from build123d import *

# Parameters (mm, degrees)
SKETCH1_R             = 10.5
SKETCH1_R_2           = 3
EXTRUDE1_DEPTH        = 46.5
SKETCH1_3_R           = 3
CUT_EXTRUDE1_DEPTH    = 49.813420286
CUT_EXTRUDE4_DEPTH    = 8.5
CUT_EXTRUDE6_START    = -37
SKETCH6_R             = 10.5
SKETCH6_R_2           = 6
CUT_EXTRUDE6_DEPTH    = 37
CUT_EXTRUDE7_START    = -1
SKETCH7_R             = 10.5
SKETCH7_R_2           = 7.5
CUT_EXTRUDE7_DEPTH    = 1
M4X0_7_TAPPED_HOLE1_D = 3
SKETCH8_OUTSIDE_W     = 33.82
SKETCH8_OUTSIDE_H     = 30.82
CUT_EXTRUDE8_DEPTH    = 30
FILLET1_R             = 0.5
CHAMFER1_SIZE         = 0.5
FILLET2_R             = 0.3
CHAMFER2_SIZE         = 1
SKETCH13_R            = 14.541098745
CUT_EXTRUDE9_DEPTH    = 9


with BuildPart() as part:
    # Sketch1 → Extrude1 (new body)
    # profile 1 of 2: a face of its own
    with BuildSketch(Plane.XY):
        Circle(SKETCH1_R)
        Circle(SKETCH1_R_2, mode=Mode.SUBTRACT)
    # profile 2 of 2: a face of its own
    with BuildSketch(Plane.XY):
        Circle(SKETCH1_R_2)
    extrude(amount=-EXTRUDE1_DEPTH)

    # Sketch1<3> → Cut-Extrude1 (cut, through all)
    with BuildSketch(Plane.XY):
        Circle(SKETCH1_3_R)
    extrude(amount=-CUT_EXTRUDE1_DEPTH, mode=Mode.SUBTRACT)

    # Sketch4 → Cut-Extrude4 (cut)
    with BuildSketch(Plane.XY):
        with BuildLine():
            Line((-10.24499878, 2.3), (10.24499878, 2.3))
            ThreePointArc((10.24499878, 2.3), (0, 10.5), (-10.24499878, 2.3))
        make_face()
    extrude(amount=-CUT_EXTRUDE4_DEPTH, mode=Mode.SUBTRACT)

    # Sketch6 → Cut-Extrude6 (cut)
    with BuildSketch(Plane(origin=(0, 0, -46.5), x_dir=(1, 0, 0), z_dir=(0, 0, -1)).offset(CUT_EXTRUDE6_START)):
        Circle(SKETCH6_R)
        with Locations(Location((0, 0, 0), (0, 0, 270))):
            Circle(SKETCH6_R_2, mode=Mode.SUBTRACT)
    extrude(amount=CUT_EXTRUDE6_DEPTH, mode=Mode.SUBTRACT)

    # Sketch7 → Cut-Extrude7 (cut)
    with BuildSketch(Plane(origin=(0, 0, -9.5), x_dir=(1, 0, 0), z_dir=(0, 0, -1)).offset(CUT_EXTRUDE7_START)):
        Circle(SKETCH7_R)
        with Locations(Location((0, 0, 0), (0, 0, 270))):
            Circle(SKETCH7_R_2, mode=Mode.SUBTRACT)
    extrude(amount=CUT_EXTRUDE7_DEPTH, mode=Mode.SUBTRACT)

    # M4x0.7 Tapped Hole1 (through all)
    with Locations(Plane(origin=(6.25, 2.3, -4.25), x_dir=(0, 0, 1), z_dir=(0, 1, 0))):
        with Locations((0, 0), (0, -12.5)):
            Hole(M4X0_7_TAPPED_HOLE1_D / 2)

    # Sketch8 outside → Cut-Extrude8 (cut)
    with BuildSketch(Plane(origin=(0, 0, -46.5), x_dir=(1, 0, 0), z_dir=(0, 0, -1))):
        with Locations((0, 1.5)):
            Rectangle(SKETCH8_OUTSIDE_W, SKETCH8_OUTSIDE_H)
        Polygon((0, 5.773502692), (-5, 2.886751346), (-5, -2.886751346), (0, -5.773502692), (5, -2.886751346), (5, 2.886751346), align=None, mode=Mode.SUBTRACT)
    extrude(amount=-CUT_EXTRUDE8_DEPTH, mode=Mode.SUBTRACT)

    # Fillet1
    fillet1_edges = [part.edges().sort_by_distance(p)[0] for p in [
        (5, -2.886751346, -31.5),
        (5, 2.886751346, -31.5),
        (0, 5.773502692, -31.5),
        (-5, 2.886751346, -31.5),
        (-5, -2.886751346, -31.5),
        (0, -5.773502692, -31.5),
    ]]
    fillet(fillet1_edges, radius=FILLET1_R)

    # Chamfer1
    chamfer1_edges = [part.edges().sort_by_distance(p)[0] for p in [
        (-2.5, -4.330127019, -46.5),
        (2.5, -4.330127019, -46.5),
        (-5, 0, -46.5),
        (-2.5, 4.330127019, -46.5),
        (2.5, 4.330127019, -46.5),
        (5, 0, -46.5),
        (0, -5.696152423, -46.5),
        (4.933012702, -2.848076211, -46.5),
        (4.933012702, 2.848076211, -46.5),
        (0, 5.696152423, -46.5),
        (-4.933012702, 2.848076211, -46.5),
        (-4.933012702, -2.848076211, -46.5),
    ]]
    chamfer(chamfer1_edges, length=CHAMFER1_SIZE - 0.0001)  # a hair under: the kernel refuses the full size

    # Sketch12 → Groove for ANSI B27.7 - 3AM1-12, Basic External Retaining Ring1 (revolve, cut)
    with BuildSketch(Plane(origin=(0, 0, 19.370057685), x_dir=(0, 1, 0), z_dir=(-1, 0, 0))):
        with BuildLine():
            Line((5.775, 33.970057685), (7.275, 33.970057685))
            Line((7.275, 33.970057685), (7.275, 35.070057685))
            Line((7.275, 35.070057685), (5.775, 35.070057685))
            ThreePointArc((5.775, 35.070057685), (5.704289322, 35.040768363), (5.675, 34.970057685))
            Line((5.675, 34.970057685), (5.675, 34.070057685))
            ThreePointArc((5.675, 34.070057685), (5.704289322, 33.999347007), (5.775, 33.970057685))
        make_face()
    revolve(axis=Axis((0, 0, 69.359173663), (0, 0, -1)), mode=Mode.SUBTRACT)

    # Fillet2
    fillet2_edges = [part.edges().sort_by_distance(p)[0] for p in [
        (0, -6, -9.5),
        (0, -7.5, -8.5),
    ]]
    fillet(fillet2_edges, radius=FILLET2_R)

    # Chamfer2
    chamfer2_edges = [part.edges().sort_by_distance(p)[0] for p in [
        (0, -10.5, 0),
        (0, -10.5, -8.5),
    ]]
    chamfer(chamfer2_edges, length=CHAMFER2_SIZE)

    # Sketch13 → Cut-Extrude9 (cut)
    with BuildSketch(Plane.XY):
        Circle(SKETCH13_R)
    extrude(amount=-CUT_EXTRUDE9_DEPTH, mode=Mode.SUBTRACT)


solid = part.part
Geometry check sheet. Reference: the model listing, model coordinates, mm. A direction names the side the tool comes from. Give positions to 0.01 mm unless a question says otherwise; leave off trailing zeros. Order: outer loops, then holes, each group sorted by start corner. A loop starts at its lowest first (then second) coordinate and runs counter-clockwise, first axis right, second up.
1) Draft check along X on faces 5 (the flat face through (-3, -1, -46.5)), 6 (the cylindrical face through (-3, 0, -27)), 7 (the cylindrical face through (-2.174, 5.242, -15.144)), 8 (the flat face through (2.35, 4.13, -46.25)). Enter one of: released by +X, released by -X, zero draft, split by the parting line, or undercut.
Results are:
face 5: zero draft
face 6: undercut
face 7: split by the parting line
face 8: released by +X
2) Cross-section at B-B (z = -37.5). Record the boundary of the cut face in (x, y), then the cut area to 3 significant figures.
Results are:
outline: (-5, -2.6) arc R0.5 ccw to (-4.75, -3.03) - (-0.25, -5.63) arc R0.5 ccw to (0.25, -5.63) - (4.75, -3.03) arc R0.5 ccw to (5, -2.6) - (5, 2.6) arc R0.5 ccw to (4.75, 3.03) - (0.25, 5.63) arc R0.5 ccw to (-0.25, 5.63) - (-4.75, 3.03) arc R0.5 ccw to (-5, 2.6) - close; hole circle Ø6 at (0, 0)
area: 58.2 mm2
3) Material ranges on probe 1 along Y at (x, z) = (0, -25); probe 2 along Y at (x, z) = (2, -43.5); probe 3 along Z at (x, y) = (-4.5, -4.5), recorded low to high.
Results are:
probe 1: y = -5.7 to -3, 3 to 5.7
probe 2: y = -4.62 to -2.24, 2.24 to 4.62
probe 3: z = -9.5 to -9
4) Tool access check on faces 1 (the flat face through (-2.469, -4.348, -31.457)), 2 (the flat face through (2.469, 4.348, -31.457)), 3 (the flat face through (-2.7, 4.4, -16.5)), 4 (the flat face through (5, 0, -31)). Record the directions out of +Z, -Z, +X, -X, +Y, -Y that give a thin tool (end or side, any length) a straight path to the whole face; none if there is none.
Results are:
face 1: -Z, -X, -Y
face 2: -Z, +X, +Y
face 3: -Z
face 4: -Z, +X, +Y, -Y
5) Gauge pin test, flat ends, axial feed: pin 1 (8 mm diameter, centred on y = -4, z = -15.5, fed in from -X); pin 2 (4 mm diameter, centred on x = 5.5, y = -5.5, fed in from -Z); pin 3 (6 mm diameter, centred on y = -1, z = -41, fed in from -X). Record the tip position at first contact, or that the pin passes through.
Results are:
pin 1: stops at x = -6
pin 2: stops at z = -16.5
pin 3: stops at x = -5
